from build123d import *

# Parameters (mm, degrees)
F0_W     = 1224
F0_H     = 400
F1_DEPTH = 2000
F2_W     = 1224
F2_H     = 1188
F3_DEPTH = 250
F4_T     = -12


# Not quite as in the source:
# - a shell that OpenCascade refuses in one call is made with other operations: the cavity is built on its own and cut out


with BuildPart() as f1:
    # F0 (on Top) → F1 (new body)
    with BuildSketch(Plane.XY):
        Rectangle(F0_W, F0_H)
    extrude(amount=F1_DEPTH)

    # F2 (on face) → F3 (cut)
    with BuildSketch(Plane.XZ.offset(200)):
        with Locations((0, 1406)):
            Rectangle(F2_W, F2_H)
    extrude(amount=-F3_DEPTH, mode=Mode.SUBTRACT)

    # F4: a shell. OpenCascade refuses it in one call, so the cavity is built on its own and cut out:
    # the body offset inwards by the wall thickness, plus a prism from it out through each open face.
    f4_core = offset(f1.part, amount=F4_T, kind=Kind.INTERSECTION, mode=Mode.PRIVATE)
    f4_exits = [f4_core.faces().sort_by_distance(p)[0] for p in [
        (0, 188, 1000),
        (0, 62, 1394),
        (0, -188, 406),
    ]]
    add(f4_core, mode=Mode.SUBTRACT)
    extrude(f4_exits, amount=-F4_T, mode=Mode.SUBTRACT)


solid = f1.part
Read the model definition and answer for the solid it produces. Units are mm, in the model's axes. A direction names the side the tool comes from. Give positions to 0.01 mm unless a question says otherwise; leave off trailing zeros. Loops run counter-clockwise (first coordinate to the right, second up) from the corner with the lowest first, then second, coordinate; pieces in that order, holes last. Notation, with made-up numbers: (6, 75) - (15, 75) arc R9 cw to (15, 89) - close; hole circle Ø1 at (68.5, 38.25). An arc over 180 degrees is marked (long way). Answer as CSV lines item,"result". Start each with the question number.
1) Find section A-A (z = 1690). Write down the section's boundary in (x, y), then the cut area to 3 significant figures.
2) Straight lines are drawn through the part: L1, parallel to Z at x = -230, y = 0.5; L2, parallel to X at y = 95, z = 759; L3, parallel to Z at x = -481.5, y = 51.5. For each, find the intervals that lie inside material, in ascending order. Write a range as from..to.
3) Determine the mould class of faces 3 (the face through (-8, 124, 1988)), 4 (the face through (-9, 126, 2000)), 5 (the face through (612, 42, 764)) for opening direction Z: released by +Z, released by -Z, zero draft, split by the parting line, or undercut.
4) Each of these flat-tipped pins is pushed along its axis until it touches: pin 1 Ø4 at (y, z) = (47.5, 1789.5) entering from +X; pin 2 Ø13 at (x, z) = (-183.5, 803.5) entering from +Y. Where does it stop, or does it pass through?
5) Find section D-D (y = 99.5). Write down the section's boundary in (x, z).
6) Find section B-B (y = -72). Write down the section's boundary in (x, z).
7) Which of the six approach directions +Z, -Z, +X, -X, +Y, -Y give full straight-line access (tool end or side, diameter ignored) to faces 1 (the face through (-9, 3, 0)), 2 (the face through (-8, -73, 800))?
8) Find section C-C (x = -107.5). Write down the section's boundary in (y, z), then the cut area to 3 significant figures.
Findings below:
1,outline,"(-612, 50) - (-600, 50) - (-600, 200) - (-612, 200) - close; (600, 50) - (612, 50) - (612, 200) - (600, 200) - close"
1,area,"3,600 mm^2"
2,L1,"0..12, 800..812"
2,L2,"-612..-600, 600..612"
2,L3,"0..12, 1988..2000"
3,face 3,"undercut"
3,face 4,"released by +Z"
3,face 5,"zero draft"
4,pin 1,"through"
4,pin 2,"y = 50"
5,outline,"(-612, 0) - (612, 0) - (612, 2000) - (-612, 2000) - close; hole (-600, 12) - (600, 12) - (600, 1988) - (-600, 1988) - close"
6,outline,"(-612, 0) - (612, 0) - (612, 812) - (-612, 812) - close; hole (-600, 12) - (600, 12) - (600, 800) - (-600, 800) - close"
7,face 1,"-Z, +X, -X, +Y, -Y"
7,face 2,"+Y, -Y"
8,outline,"(-200, 0) - (200, 0) - (200, 12) - (-200, 12) - close; (-200, 800) - (50, 800) - (50, 812) - (-200, 812) - close; (50, 1988) - (200, 1988) - (200, 2000) - (50, 2000) - close"
8,area,"9,600 mm^2"
